Source: CAD feature listing. Evaluate the final solid. Frame: model axes, mm. A direction names the side the tool comes from. Round coordinates to 2 decimals unless told otherwise and drop trailing zeros. Loops run counter-clockwise (first coordinate to the right, second up) from the corner with the lowest first, then second, coordinate; pieces in that order, holes last. Notation, with made-up numbers: (-30.75, 21) - (-4.75, 21) arc R22 ccw to (-4.75, 32) - close; hole circle Ø7 at (41, -34). An arc over 180 degrees is marked (long way). Write item = value, one per line. Start each with the question number.
from build123d import *

# Parameters (mm, degrees)
F1_DEPTH = 190.5
F2_R     = 10.818044
F3_DEPTH = 127
F2_R_2   = 10.691628
F4_DEPTH = 127
F5_R     = 11.141962
F5_R_2   = 10.916341
F6_DEPTH = 76.2
F7_R     = 10.875838
F8_DEPTH = 76.2


with BuildPart() as f1:
    # F0 (on Right) → F1 (new body)
    with BuildSketch(Plane.YZ):
        with BuildLine():
            ThreePointArc((-79.597275, 10.571338), (-85.746525, -5.640093), (-68.586435, -8.121035))
            ThreePointArc((-68.586435, -8.121035), (-66.596902, 5.640093), (-79.597275, 10.571338))
        make_face()
    extrude(amount=F1_DEPTH)

    # F2 (on Top) → F3 (join)
    with BuildSketch(Plane.XY):
        with Locations((0, -76.424129)):
            Circle(F2_R)
    extrude(amount=F3_DEPTH)

    # F2 (on Top) → F4 (join)
    with BuildSketch(Plane.XY):
        with Locations((0, -76.424129)):
            Circle(F2_R)
        with Locations((190.621048, -76.424129)):
            Circle(F2_R_2)
    extrude(amount=F4_DEPTH)

    # F5 (on Right) → F6 (join)
    with BuildSketch(Plane.YZ):
        with Locations((-76.848619, 115.551263)):
            Circle(F5_R)
        with Locations((-76.848619, 115.551263)):
            Circle(F5_R_2, mode=Mode.SUBTRACT)
    extrude(amount=-F6_DEPTH)

    # F7 (on face) → F8 (join)
    with BuildSketch(Plane.YZ.offset(190.5)):
        with Locations((-76.119892, 116.334341)):
            Circle(F7_R)
    extrude(amount=F8_DEPTH)


solid = f1.part
(1) Access query for faces 4 (the face through (195, -76, 0)), 5 (the face through (266.7, -76, 116)), 6 (the face through (-8.58, -83.01, 62.61)), 7 (the face through (228.067, -70.273, 125.505)). Directions: +Z, -Z, +X, -X, +Y, -Y. A direction counts if a zero-diameter tool reaches every point of the face in a straight line with its end or side. Return the directions, or none.
(2) Cut plane C-C (x = 112.5). Output: boundary loops of the cut face in (y, z) (1 decimal), and give its area (3 significant figures).
(3) Cut plane B-B (z = 68.5). Output: boundary loops of the cut face in (x, y).
(4) Mould query, pull axis Y, two halves, no side actions, for faces 1 (the face through (-37.6, -78.3, 126.6)), 2 (the face through (-4, -76, 0)), 3 (the face through (-37.567, -87.754, 116.031)). Classes: +Y half, -Y half, draft (parallel to the pull), parting line (faces both ways), or undercut.
(5) Cut plane A-A (x = -7). Output: boundary loops of the cut face in (y, z).
(6) Material intervals for line 1 along X through (y, z) = (-76.5, 91.5); line 2 along X through (y, z) = (-70.5, -3); line 3 along X through (y, z) = (-84, 110), sorted ascending. Write a range as from..to.
(7) Pin query (flat end, axial travel): P1, Ø4, axis at y = -77, z = 21, coming from the -X side; P2, Ø12, axis at x = 14.5, z = 55.5, coming from the +Y side; P3, Ø7.5, axis at y = -73, z = -4, coming from the +X side. Return the tip coordinate at first contact, or that it passes through.
Solution:
q1.face_4 = -Z, +X, +Y, -Y
q1.face_5 = +Z, -Z, +X, +Y, -Y
q1.face_6 = none
q1.face_7 = +X
q2.outline = circle Ø22.2 at (-76.2, 0)
q2.area = 388 mm^2
q3.outline = circle Ø21.64 at (0, -76.42); circle Ø21.38 at (190.62, -76.42)
q4.face_1 = parting line
q4.face_2 = draft
q4.face_3 = undercut
q5.outline = (-84.67, 0) - (-68.18, 0) - (-68.18, 108.56) arc R11.14 ccw to (-68.18, 122.55) - (-68.18, 127) - (-84.67, 127) - (-84.67, 123.48) arc R11.14 ccw to (-84.67, 107.62) - close; hole (-84.67, 107.94) - (-84.67, 123.16) arc R10.92 ccw to start; hole (-68.18, 108.92) arc R10.92 ccw to (-68.18, 122.18) - close
q6.line_1 = -10.82..10.82, 179.93..201.31
q6.line_2 = 0..190.5
q6.line_3 = -7.72..7.72, 183.08..266.7
q7.P1 = -10.82
q7.P2 = -69.73
q7.P3 = 190.5
